```python
from build123d import *

# Parameters (mm, degrees)
F2_W     = 10
F2_H     = 10.684083
F3_DEPTH = 40.5
F4_SIZE  = 2


with BuildPart() as f1:
    # F0 (on Front) → F1 (revolve)
    with BuildSketch(Plane.XZ):
        with BuildLine():
            ThreePointArc((-6.349949, -3.617726), (-20.37432, 8.030333), (-26.638337, 25.151149))
            Line((-26.638337, 25.151149), (-27.5, 35))
            Line((-27.5, 35), (-29, 35))
            Line((-29, 35), (-29, 30))
            Line((-29, 30), (-30.074017, 30))
            Line((-30.074017, 30), (-29.626922, 24.889682))
            ThreePointArc((-29.626922, 24.889682), (-26.737592, 13.322956), (-20.406444, 3.220781))
            ThreePointArc((-20.406444, 3.220781), (-19.232291, -0.826148), (-21.56813, -4.333301))
            Line((-21.56813, -4.333301), (-27.557738, -7.991337))
            ThreePointArc((-27.557738, -7.991337), (-29.31231, -9.812077), (-29.951671, -12.258469))
            Line((-29.951671, -12.258469), (-29.951671, -14))
            Line((-29.951671, -14), (-28.951671, -15))
            Line((-28.951671, -15), (0, -15))
            Line((0, -15), (0, -4.52649))
            Line((0, -4.52649), (-2.184685, -4.52649))
            ThreePointArc((-2.184685, -4.52649), (-4.316309, -4.296658), (-6.349949, -3.617726))
        make_face()
    revolve(axis=Axis((0, 0, -9.763245), (0, 0, -1)))

    # F2 (on Front) → F3 (cut, symmetric)
    with BuildSketch(Plane.XZ):
        with Locations((0, -15.342041)):
            Rectangle(F2_W, F2_H)
    extrude(amount=F3_DEPTH, both=True, mode=Mode.SUBTRACT)

    # F4
    f4_edges = [f1.edges().sort_by_distance(p)[0] for p in [
        (-5, 0, -10),
        (5, 0, -10),
    ]]
    chamfer(f4_edges, length=F4_SIZE)


solid = f1.part
```
Build history of the part. All positions in model axes, mm. A direction names the side the tool comes from. Round coordinates to 2 decimals unless told otherwise and drop trailing zeros. Write each loop counter-clockwise with the first axis right and the second up, starting at its lowest first coordinate (ties: lowest second). Pieces come first, ordered by that corner, then holes. Notation, with made-up numbers: (0, 63) -> (50, 63) arc R17 cw to (50, 80) -> close; hole circle Ø3 at (-2, 1). An arc over 180 degrees is marked (long way). Put each result on its own line as item: value.
Item 1: Wall check: probe 1 along Y at (x, z) = (-8, -10.5); probe 2 along Y at (x, z) = (-3.5, 9); probe 3 along Y at (x, z) = (-5, -2.5). Give the ranges that are in metal, low to high. Write a range as from..to.
Here are the results:
probe 1: y = -28.53..28.53
probe 2: y = -24.31..-20.74, 20.74..24.31
probe 3: y = -19.17..-6.97, 6.97..19.17
Item 2: Flat gauge pins, fed straight in: P1, Ø5, axis at y = 6.5, z = 10, coming from the -X side; P2, Ø12, axis at y = 17, z = 25.5, coming from the -X side; P3, Ø2, axis at x = -0.5, y = -0.5, coming from the +Z side. Where does each tip first touch, or does it go through?
Here are the results:
P1: stops at x = -25.7
P2: stops at x = -27.63
P3: stops at z = -4.53
Item 3: Slice it at A-A, the plane z = 31.5. Give the cut face in (x, y), plus the area to 3 significant figures.
Here are the results:
outline: circle Ø58 at (0, 0); hole circle Ø54.39 at (0, 0)
area: 319 mm^2
Item 4: Tool access for faces 1 (the face through (-10.125, -19.467, -4.562)), 2 (the face through (29.946, 0.588, -13.141)), 3 (the face through (0, 0, -10)), 4 (the face through (-13.38, -25.73, 32.47)): list every direction of +Z, -Z, +X, -X, +Y, -Y with a clear straight run to the whole face (end or side of a thin tool).
Here are the results:
face 1: none
face 2: -Z, +X
face 3: -Z, +Y, -Y
face 4: +Z
Item 5: Two-plate mould, pull along X, no slides. Class faces 5 (the face through (-5, 0, -14)), 6 (the face through (-29.946, -0.588, -13.141)), 7 (the face through (6.427, -28.944, 25.138)): pulls with the +X half, pulls with the -X half, needs draft (parallel to the pull), parting line crosses it, or undercut.
Here are the results:
face 5: undercut
face 6: pulls with the -X half
face 7: parting line crosses it
